The listing builds one solid part. Answer for the finished solid, in the listing's coordinates (mm). A direction names the side the tool comes from. Round coordinates to 2 decimals unless told otherwise and drop trailing zeros. Write each loop counter-clockwise with the first axis right and the second up, starting at its lowest first coordinate (ties: lowest second). Pieces come first, ordered by that corner, then holes.
(1) Find the intervals of material crossed by probe 1 along X at (y, z) = (-1, 0); probe 2 along Z at (x, y) = (-490, 8); probe 3 along X at (y, z) = (21, -2), in increasing order.
(2) For faces 5 (the face through (-475, -16, -16)), 6 (the face through (-490, 0, 20)), 7 (the face through (-500, -20, -5)), determine the directions among +Z, -Z, +X, -X, +Y, -Y from which every point of the face is accessible in a straight line to the end or side of a thin tool.
(3) Each of these flat-tipped pins is pushed along its axis until it touches: pin 1 Ø6 at (x, y) = (380.5, 7.5) entering from -Z; pin 2 Ø5 at (x, z) = (-12, -3.5) entering from -Y (3 decimals); pin 3 Ø17.5 at (x, z) = (-490, 0) entering from +Y; pin 4 Ø8 at (x, z) = (-67, -11) entering from +Y (3 decimals). Where does it stop, or does it pass through?
(4) The mould has two halves that part along X. Classify faces 1 (the face through (-490, 0, -20)), 2 (the face through (555, 0, 0)), 3 (the face through (-475, 16, 15)), 4 (the face through (-475, -15, 16)): +X half, -X half, draft (parallel to the pull), parting line (faces both ways), or undercut.
(5) A cutting plane is placed at A-A, the plane x = -490. Give the vertices of the cut face in (y, z), and give its area (3 significant figures).
from build123d import *

# Parameters (mm, degrees)
F0_R          = 20
F1_DEPTH      = 505
F2_R          = 25
F2_R_2        = 20
F1_FACE_R     = 20
F3_DEPTH      = 50
F2_R_3        = 32.5
F4_DEPTH      = 15
F5_R          = 11
F6_DEPTH      = 32.501
F6_DEPTH_BACK = 25
F8_DEPTH      = 30
F10_DEPTH     = 52.501


with BuildPart() as f1:
    # F0 (on Right) → F1 (new body, symmetric)
    with BuildSketch(Plane.YZ):
        Circle(F0_R)
    extrude(amount=F1_DEPTH, both=True)

    # F2 (on face) + F1_face (on face) → F3 (join)
    with BuildSketch(Plane.YZ.offset(505)):
        Circle(F2_R)
        Circle(F2_R_2, mode=Mode.SUBTRACT)
    with BuildSketch(Plane.YZ.offset(505)):
        Circle(F1_FACE_R)
    extrude(amount=F3_DEPTH)

    # F2 (on face) → F4 (join)
    with BuildSketch(Plane.YZ.offset(505)):
        Circle(F2_R_3)
        Circle(F2_R, mode=Mode.SUBTRACT)
    extrude(amount=F4_DEPTH)

    # F5 (on Front) → F6 (cut, two sides)
    with BuildSketch(Plane.XZ) as f6_sk:
        with Locations((-490, 0)):
            Circle(F5_R)
    extrude(amount=-F6_DEPTH, mode=Mode.SUBTRACT)
    extrude(f6_sk.sketch, amount=F6_DEPTH_BACK, mode=Mode.SUBTRACT)

    # F7 (on face) → F8 (join)
    with BuildSketch(Plane(origin=(-505, 0, 0), x_dir=(0, -1, 0), z_dir=(-1, 0, 0))):
        with BuildLine():
            ThreePointArc((-20, 0), (-14.1421356364, 14.142135611), (-3.59e-08, 20))
            Line((-3.59e-08, 20), (-20, 20))
            Line((-20, 20), (-20, 0))
        make_face()
        with BuildLine():
            ThreePointArc((0, -20), (-14.1421356237, -14.1421356237), (-20, 0))
            Line((-20, 0), (-20, -20))
            Line((-20, -20), (0, -20))
        make_face()
        with BuildLine():
            Line((20, -20), (20, 0))
            ThreePointArc((20, 0), (14.1421356237, -14.1421356237), (0, -20))
            Line((0, -20), (20, -20))
        make_face()
        with BuildLine():
            Line((20, 0), (20, 20))
            Line((20, 20), (-3.59e-08, 20))
            ThreePointArc((-3.59e-08, 20), (14.142135611, 14.1421356364), (20, 0))
        make_face()
    extrude(amount=-F8_DEPTH)

    # F9 (on face) → F10 (cut, through all)
    with BuildSketch(Plane.XZ.offset(20)):
        with BuildLine():
            Line((-501, 0), (-479, 0))
            ThreePointArc((-479, 0), (-490, 11), (-501, 0))
        make_face()
        with BuildLine():
            ThreePointArc((-501, 0), (-490, -11), (-479, 0))
            Line((-479, 0), (-501, 0))
        make_face()
    extrude(amount=-F10_DEPTH, mode=Mode.SUBTRACT)


solid = f1.part
Solutions:
1. probe 1: x = -505 to -501, -479 to 555
1. probe 2: z = -20 to -11, 11 to 20
1. probe 3: x = 505 to 555
2. face 5: -Z, -Y
2. face 6: +Z, -X, +Y, -Y
2. face 7: +Z, -Z, -X, -Y
3. pin 1: stops at z = -19.49
3. pin 2: stops at y = -19.975
3. pin 3: passes through
3. pin 4: stops at y = 18.735
4. face 1: draft
4. face 2: +X half
4. face 3: undercut
4. face 4: undercut
5. outline: (-20, -20) - (20, -20) - (20, -11) - (-20, -11) - close; (-20, 11) - (20, 11) - (20, 20) - (-20, 20) - close
5. area: 720 mm2
